Geometry: final body of the model. Coordinates: model frame, mm. A direction names the side the tool comes from. Give positions to 0.01 mm unless a question says otherwise; leave off trailing zeros. Write each loop counter-clockwise with the first axis right and the second up, starting at its lowest first coordinate (ties: lowest second). Pieces come first, ordered by that corner, then holes. Notation, with made-up numbers: M 45,73.5 L 76,73.5 A18 ccw 76,97.5 Z; hole C 28.5,24.25 d5. An arc over 180 degrees is marked long. Use a Markdown table: item, result. Add a question column.
1) Line query: line 1 (X direction, y = 7.75, z = 12.5); line 2 (Z direction, x = 4, y = -4.75); line 3 (Y direction, x = -0.25, z = 12.75). Output: solid intervals per line, ascending.
2) Section C-C on z = 21.25. Return the cut outline in (x, y), then the cut area to 3 significant figures.
3) Pin query (flat end, axial travel): pin 1 (3 mm diameter, centred on x = -8.5, y = -5.5, fed in from +Z); pin 2 (5 mm diameter, centred on x = 4.5, y = -3.5, fed in from +Z); pin 3 (5 mm diameter, centred on x = -4, z = 8.5, fed in from -Y); pin 4 (8 mm diameter, centred on y = -5.5, z = 16, fed in from -X). Return the tip coordinate at first contact, or that it passes through.
4) Draft query along X for faces 6 (the cylindrical face through (-1.19, -5.37, 19.44)), 7 (the cylindrical face through (-7.485, 6.448, 6.619)), 8 (the cylindrical face through (-3.393, 10.463, 6.619)), 9 (the cylindrical face through (3.393, -10.463, 6.619)). Return one class per face: +X half, -X half, draft (parallel to the pull), parting line (faces both ways), or undercut.
5) Section A-A on y = 0. Return the cut outline in (x, z), then the cut area to 3 significant figures.
6) Set-up query: faces 1 (the cylindrical face through (10.463, 3.393, 6.619)), 2 (the cylindrical face through (-9.616, -2.265, 6.619)), 3 (the cylindrical face through (5.152, 8.467, 6.619)), 4 (the cylindrical face through (3.82, -9.14, 6.62)), 5 (the cylindrical face through (-0.817, -9.846, 6.619)). Return all of +Z, -Z, +X, -X, +Y, -Y with unobstructed straight access to the full face (end or side cutting, diameter ignored); none if empty.
```python
from build123d import *

# Parameters (mm, degrees)
AUFSATZ_LINEAR_AUSTRAGEN1_DEPTH = 17
SKIZZE2_R                       = 5.5
AUFSATZ_LINEAR_AUSTRAGEN3_DEPTH = 10
FASE1_SIZE                      = 1


with BuildPart() as part:
    # Skizze1 → Aufsatz-Linear austragen1 (new body)
    with BuildSketch(Plane.XY.offset(14.999999972)):
        with BuildLine():
            ThreePointArc((-1.707040323, 8.581871229), (-2.274158717, 9.63053951), (-2.985844941, 10.587007573))
            ThreePointArc((-2.985844941, 10.587007573), (-3.399186929, 10.461621652), (-3.807287618, 10.320104668))
            ThreePointArc((-3.807287618, 10.320104668), (-3.820856046, 9.127987084), (-3.663272714, 7.946252795))
            ThreePointArc((-3.663272714, 7.946252795), (-3.972416885, 7.79630711), (-4.275435876, 7.634340085))
            ThreePointArc((-4.275435876, 7.634340085), (-5.138853841, 8.456433665), (-6.111272547, 9.146165711))
            ThreePointArc((-6.111272547, 9.146165711), (-6.465637758, 8.899186915), (-6.810033424, 8.638486217))
            ThreePointArc((-6.810033424, 8.638486217), (-6.454553173, 7.500522146), (-5.939506541, 6.425321977))
            ThreePointArc((-5.939506541, 6.425321977), (-6.187184354, 6.187184354), (-6.425321977, 5.939506541))
            ThreePointArc((-6.425321977, 5.939506541), (-7.500522146, 6.454553173), (-8.638486217, 6.810033424))
            ThreePointArc((-8.638486217, 6.810033424), (-8.899186915, 6.465637758), (-9.146165711, 6.111272547))
            ThreePointArc((-9.146165711, 6.111272547), (-8.456433665, 5.138853841), (-7.634340085, 4.275435876))
            ThreePointArc((-7.634340085, 4.275435876), (-7.79630711, 3.972416885), (-7.946252795, 3.663272714))
            ThreePointArc((-7.946252795, 3.663272714), (-9.127987084, 3.820856046), (-10.320104668, 3.807287618))
            ThreePointArc((-10.320104668, 3.807287618), (-10.461621652, 3.399186929), (-10.587007573, 2.985844941))
            ThreePointArc((-10.587007573, 2.985844941), (-9.63053951, 2.274158717), (-8.581871229, 1.707040323))
            ThreePointArc((-8.581871229, 1.707040323), (-8.642273006, 1.368801573), (-8.689349024, 1.028452231))
            ThreePointArc((-8.689349024, 1.028452231), (-9.861941048, 0.813146907), (-10.99151937, 0.431857972))
            ThreePointArc((-10.99151937, 0.431857972), (-10.999999971, 0), (-10.99151937, -0.431857972))
            ThreePointArc((-10.99151937, -0.431857972), (-9.861941048, -0.813146907), (-8.689349024, -1.028452231))
            ThreePointArc((-8.689349024, -1.028452231), (-8.642273006, -1.368801573), (-8.581871229, -1.707040323))
            ThreePointArc((-8.581871229, -1.707040323), (-9.63053951, -2.274158717), (-10.587007573, -2.985844941))
            ThreePointArc((-10.587007573, -2.985844941), (-10.461621652, -3.399186929), (-10.320104668, -3.807287618))
            ThreePointArc((-10.320104668, -3.807287618), (-9.127987084, -3.820856046), (-7.946252795, -3.663272714))
            ThreePointArc((-7.946252795, -3.663272714), (-7.79630711, -3.972416885), (-7.634340085, -4.275435876))
            ThreePointArc((-7.634340085, -4.275435876), (-8.456433665, -5.138853841), (-9.146165711, -6.111272547))
            ThreePointArc((-9.146165711, -6.111272547), (-8.899186915, -6.465637758), (-8.638486217, -6.810033424))
            ThreePointArc((-8.638486217, -6.810033424), (-7.500522146, -6.454553173), (-6.425321977, -5.939506541))
            ThreePointArc((-6.425321977, -5.939506541), (-6.187184354, -6.187184354), (-5.939506541, -6.425321977))
            ThreePointArc((-5.939506541, -6.425321977), (-6.454553173, -7.500522146), (-6.810033424, -8.638486217))
            ThreePointArc((-6.810033424, -8.638486217), (-6.465637758, -8.899186915), (-6.111272547, -9.146165711))
            ThreePointArc((-6.111272547, -9.146165711), (-5.138853841, -8.456433665), (-4.275435876, -7.634340085))
            ThreePointArc((-4.275435876, -7.634340085), (-3.972416885, -7.79630711), (-3.663272714, -7.946252795))
            ThreePointArc((-3.663272714, -7.946252795), (-3.820856046, -9.127987084), (-3.807287618, -10.320104668))
            ThreePointArc((-3.807287618, -10.320104668), (-3.399186929, -10.461621652), (-2.985844941, -10.587007573))
            ThreePointArc((-2.985844941, -10.587007573), (-2.274158717, -9.63053951), (-1.707040323, -8.581871229))
            ThreePointArc((-1.707040323, -8.581871229), (-1.368801573, -8.642273006), (-1.028452231, -8.689349024))
            ThreePointArc((-1.028452231, -8.689349024), (-0.813146907, -9.861941048), (-0.431857972, -10.99151937))
            ThreePointArc((-0.431857972, -10.99151937), (0, -10.999999971), (0.431857972, -10.99151937))
            ThreePointArc((0.431857972, -10.99151937), (0.813146907, -9.861941048), (1.028452231, -8.689349024))
            ThreePointArc((1.028452231, -8.689349024), (1.368801573, -8.642273006), (1.707040323, -8.581871229))
            ThreePointArc((1.707040323, -8.581871229), (2.274158717, -9.63053951), (2.985844941, -10.587007573))
            ThreePointArc((2.985844941, -10.587007573), (3.399186929, -10.461621652), (3.807287618, -10.320104668))
            ThreePointArc((3.807287618, -10.320104668), (3.820856046, -9.127987084), (3.663272714, -7.946252795))
            ThreePointArc((3.663272714, -7.946252795), (3.972416885, -7.79630711), (4.275435876, -7.634340085))
            ThreePointArc((4.275435876, -7.634340085), (5.138853841, -8.456433665), (6.111272547, -9.146165711))
            ThreePointArc((6.111272547, -9.146165711), (6.465637758, -8.899186915), (6.810033424, -8.638486217))
            ThreePointArc((6.810033424, -8.638486217), (6.454553173, -7.500522146), (5.939506541, -6.425321977))
            ThreePointArc((5.939506541, -6.425321977), (6.187184354, -6.187184354), (6.425321977, -5.939506541))
            ThreePointArc((6.425321977, -5.939506541), (7.500522146, -6.454553173), (8.638486217, -6.810033424))
            ThreePointArc((8.638486217, -6.810033424), (8.899186915, -6.465637758), (9.146165711, -6.111272547))
            ThreePointArc((9.146165711, -6.111272547), (8.456433665, -5.138853841), (7.634340085, -4.275435876))
            ThreePointArc((7.634340085, -4.275435876), (7.79630711, -3.972416885), (7.946252795, -3.663272714))
            ThreePointArc((7.946252795, -3.663272714), (9.127987084, -3.820856046), (10.320104668, -3.807287618))
            ThreePointArc((10.320104668, -3.807287618), (10.461621652, -3.399186929), (10.587007573, -2.985844941))
            ThreePointArc((10.587007573, -2.985844941), (9.63053951, -2.274158717), (8.581871229, -1.707040323))
            ThreePointArc((8.581871229, -1.707040323), (8.642273006, -1.368801573), (8.689349024, -1.028452231))
            ThreePointArc((8.689349024, -1.028452231), (9.861941048, -0.813146907), (10.99151937, -0.431857972))
            ThreePointArc((10.99151937, -0.431857972), (10.999999971, 0), (10.99151937, 0.431857972))
            ThreePointArc((10.99151937, 0.431857972), (9.861941048, 0.813146907), (8.689349024, 1.028452231))
            ThreePointArc((8.689349024, 1.028452231), (8.642273006, 1.368801573), (8.581871229, 1.707040323))
            ThreePointArc((8.581871229, 1.707040323), (9.63053951, 2.274158717), (10.587007573, 2.985844941))
            ThreePointArc((10.587007573, 2.985844941), (10.461621652, 3.399186929), (10.320104668, 3.807287618))
            ThreePointArc((10.320104668, 3.807287618), (9.127987084, 3.820856046), (7.946252795, 3.663272714))
            ThreePointArc((7.946252795, 3.663272714), (7.79630711, 3.972416885), (7.634340085, 4.275435876))
            ThreePointArc((7.634340085, 4.275435876), (8.456433665, 5.138853841), (9.146165711, 6.111272547))
            ThreePointArc((9.146165711, 6.111272547), (8.899186915, 6.465637758), (8.638486217, 6.810033424))
            ThreePointArc((8.638486217, 6.810033424), (7.500522146, 6.454553173), (6.425321977, 5.939506541))
            ThreePointArc((6.425321977, 5.939506541), (6.187184354, 6.187184354), (5.939506541, 6.425321977))
            ThreePointArc((5.939506541, 6.425321977), (6.454553173, 7.500522146), (6.810033424, 8.638486217))
            ThreePointArc((6.810033424, 8.638486217), (6.465637758, 8.899186915), (6.111272547, 9.146165711))
            ThreePointArc((6.111272547, 9.146165711), (5.138853841, 8.456433665), (4.275435876, 7.634340085))
            ThreePointArc((4.275435876, 7.634340085), (3.972416885, 7.79630711), (3.663272714, 7.946252795))
            ThreePointArc((3.663272714, 7.946252795), (3.820856046, 9.127987084), (3.807287618, 10.320104668))
            ThreePointArc((3.807287618, 10.320104668), (3.399186929, 10.461621652), (2.985844941, 10.587007573))
            ThreePointArc((2.985844941, 10.587007573), (2.274158717, 9.63053951), (1.707040323, 8.581871229))
            ThreePointArc((1.707040323, 8.581871229), (1.368801573, 8.642273006), (1.028452231, 8.689349024))
            ThreePointArc((1.028452231, 8.689349024), (0.813146907, 9.861941048), (0.431857972, 10.99151937))
            ThreePointArc((0.431857972, 10.99151937), (0, 10.999999971), (-0.431857972, 10.99151937))
            ThreePointArc((-0.431857972, 10.99151937), (-0.813146907, 9.861941048), (-1.028452231, 8.689349024))
            ThreePointArc((-1.028452231, 8.689349024), (-1.368801573, 8.642273006), (-1.707040323, 8.581871229))
        make_face()
    extrude(amount=-AUFSATZ_LINEAR_AUSTRAGEN1_DEPTH)

    # Skizze2 → Aufsatz-Linear austragen3 (add)
    with BuildSketch(Plane.XY.offset(14.999999972)):
        Circle(SKIZZE2_R)
    extrude(amount=AUFSATZ_LINEAR_AUSTRAGEN3_DEPTH)

    # Fase1
    fase1_edges = [part.edges().sort_by_distance(p)[0] for p in [
        (-5.5, 0, 24.999999972),
    ]]
    chamfer(fase1_edges, length=FASE1_SIZE)


solid = part.part
```
Found:
| question | item | result |
|---|---|---|
| 1 | line 1 | -6.55 to -4.38, -4.06 to 4.06, 4.38 to 6.55 |
| 1 | line 2 | -2 to 15 |
| 1 | line 3 | -11 to 11 |
| 2 | outline | C 0,0 d11 |
| 2 | area | 95.0 mm² |
| 3 | pin 1 | z = 15 |
| 3 | pin 2 | z = 25 |
| 3 | pin 3 | y = -10.59 |
| 3 | pin 4 | x = -10.59 |
| 4 | face 6 | parting line |
| 4 | face 7 | undercut |
| 4 | face 8 | -X half |
| 4 | face 9 | +X half |
| 5 | outline | M -11,-2 L 11,-2 L 11,15 L 5.5,15 L 5.5,24 L 4.5,25 L -4.5,25 L -5.5,24 L -5.5,15 L -11,15 Z |
| 5 | area | 483 mm² |
| 6 | face 1 | +Z, -Z, +X, +Y |
| 6 | face 2 | +Z, -Z, -X |
| 6 | face 3 | +Z, -Z, +Y |
| 6 | face 4 | +Z, -Z |
| 6 | face 5 | +Z, -Z, -Y |
